from build123d import *

# Parameters (mm, degrees)
SKETCH1_R           = 1.6
SKETCH1_R_2         = 1.65
BOSS_EXTRUDE1_DEPTH = 4
FILLET2_R           = 10
FILLET3_R           = 5


with BuildPart() as part:
    # Sketch1 → Boss-Extrude1 (new body)
    with BuildSketch(Plane.XY):
        with BuildLine():
            Line((1.40773023, -0.063608297), (20.206941284, -0.063608297))
            ThreePointArc((20.206941284, -0.063608297), (20.914048066, -0.356501516), (21.206941284, -1.063608297))
            Line((21.206941284, -1.063608297), (21.206941284, -3.063608297))
            ThreePointArc((21.206941284, -3.063608297), (21.499834503, -3.770715079), (22.206941284, -4.063608297))
            Line((22.206941284, -4.063608297), (72.208519176, -4.063608297))
            ThreePointArc((72.208519176, -4.063608297), (72.915625957, -3.770715079), (73.208519176, -3.063608297))
            Line((73.208519176, -3.063608297), (73.208519176, -1.063608297))
            ThreePointArc((73.208519176, -1.063608297), (73.501412395, -0.356501516), (74.208519176, -0.063608297))
            Line((74.208519176, -0.063608297), (93.00773023, -0.063608297))
            Line((93.00773023, -0.063608297), (93.00773023, 19.936391703))
            Line((93.00773023, 19.936391703), (72.20773023, 31.430017028))
            Line((72.20773023, 31.430017028), (72.20773023, 94.442766377))
            Line((72.20773023, 94.442766377), (93.00773023, 105.936391703))
            Line((93.00773023, 105.936391703), (93.00773023, 125.936391703))
            Line((93.00773023, 125.936391703), (74.208519176, 125.936391703))
            ThreePointArc((74.208519176, 125.936391703), (73.501412395, 126.229284921), (73.208519176, 126.936391703))
            Line((73.208519176, 126.936391703), (73.208519176, 128.936391703))
            ThreePointArc((73.208519176, 128.936391703), (72.915625957, 129.643498484), (72.208519176, 129.936391703))
            Line((72.208519176, 129.936391703), (22.206941284, 129.936391703))
            ThreePointArc((22.206941284, 129.936391703), (21.499834503, 129.643498484), (21.206941284, 128.936391703))
            Line((21.206941284, 128.936391703), (21.206941284, 126.936391703))
            ThreePointArc((21.206941284, 126.936391703), (20.914048066, 126.229284921), (20.206941284, 125.936391703))
            Line((20.206941284, 125.936391703), (1.40773023, 125.936391703))
            Line((1.40773023, 125.936391703), (1.40773023, 105.936391703))
            Line((1.40773023, 105.936391703), (22.20773023, 94.442766377))
            Line((22.20773023, 94.442766377), (22.20773023, 31.430017028))
            Line((22.20773023, 31.430017028), (1.40773023, 19.936391703))
            Line((1.40773023, 19.936391703), (1.40773023, -0.063608297))
        make_face()
        with Locations((5.55773023, 4.936391703)):
            Circle(SKETCH1_R, mode=Mode.SUBTRACT)
        with Locations((14.05773023, 4.936391703)):
            Circle(SKETCH1_R, mode=Mode.SUBTRACT)
        with Locations((14.05773023, 14.936391703)):
            Circle(SKETCH1_R, mode=Mode.SUBTRACT)
        with Locations((5.55773023, 14.936391703)):
            Circle(SKETCH1_R, mode=Mode.SUBTRACT)
        with Locations(Location((69.208519176, 2.936391703, 0), (0, 0, 180))):
            Circle(SKETCH1_R, mode=Mode.SUBTRACT)
        with Locations((47.206941284, 2.936391703)):
            Circle(SKETCH1_R, mode=Mode.SUBTRACT)
        with Locations(Location((66.20773023, 54.936391703, 0), (0, 0, 180))):
            Circle(SKETCH1_R_2, mode=Mode.SUBTRACT)
        with Locations(Location((88.85773023, 14.936391703, 0), (0, 0, 180))):
            Circle(SKETCH1_R, mode=Mode.SUBTRACT)
        with Locations(Location((80.35773023, 14.936391703, 0), (0, 0, 180))):
            Circle(SKETCH1_R, mode=Mode.SUBTRACT)
        with Locations(Location((80.35773023, 4.936391703, 0), (0, 0, 180))):
            Circle(SKETCH1_R, mode=Mode.SUBTRACT)
        with Locations(Location((88.85773023, 4.936391703, 0), (0, 0, 180))):
            Circle(SKETCH1_R, mode=Mode.SUBTRACT)
        with Locations((28.20773023, 54.936391703)):
            Circle(SKETCH1_R_2, mode=Mode.SUBTRACT)
        with Locations((25.206941284, 2.936391703)):
            Circle(SKETCH1_R, mode=Mode.SUBTRACT)
        with Locations(Location((25.206941284, 122.936391703, 0), (0, 0, 180))):
            Circle(SKETCH1_R, mode=Mode.SUBTRACT)
        with Locations(Location((28.20773023, 70.936391703, 0), (0, 0, 180))):
            Circle(SKETCH1_R_2, mode=Mode.SUBTRACT)
        with Locations((88.85773023, 120.936391703)):
            Circle(SKETCH1_R, mode=Mode.SUBTRACT)
        with Locations((80.35773023, 120.936391703)):
            Circle(SKETCH1_R, mode=Mode.SUBTRACT)
        with Locations((80.35773023, 110.936391703)):
            Circle(SKETCH1_R, mode=Mode.SUBTRACT)
        with Locations((88.85773023, 110.936391703)):
            Circle(SKETCH1_R, mode=Mode.SUBTRACT)
        with Locations((66.20773023, 70.936391703)):
            Circle(SKETCH1_R_2, mode=Mode.SUBTRACT)
        with Locations(Location((47.206941284, 122.936391703, 0), (0, 0, 180))):
            Circle(SKETCH1_R, mode=Mode.SUBTRACT)
        with Locations((69.208519176, 122.936391703)):
            Circle(SKETCH1_R, mode=Mode.SUBTRACT)
        with Locations(Location((5.55773023, 110.936391703, 0), (0, 0, 180))):
            Circle(SKETCH1_R, mode=Mode.SUBTRACT)
        with Locations(Location((14.05773023, 110.936391703, 0), (0, 0, 180))):
            Circle(SKETCH1_R, mode=Mode.SUBTRACT)
        with Locations(Location((14.05773023, 120.936391703, 0), (0, 0, 180))):
            Circle(SKETCH1_R, mode=Mode.SUBTRACT)
        with Locations(Location((5.55773023, 120.936391703, 0), (0, 0, 180))):
            Circle(SKETCH1_R, mode=Mode.SUBTRACT)
    extrude(amount=BOSS_EXTRUDE1_DEPTH)

    # Fillet2
    fillet2_edges = [part.edges().sort_by_distance(p)[0] for p in [
        (1.40773023, 19.936391703, 2),
        (22.20773023, 31.430017028, 2),
        (22.20773023, 94.442766377, 2),
        (1.40773023, 105.936391703, 2),
        (93.00773023, 105.936391703, 2),
        (72.20773023, 94.442766377, 2),
        (72.20773023, 31.430017028, 2),
        (93.00773023, 19.936391703, 2),
    ]]
    fillet(fillet2_edges, radius=FILLET2_R)

    # Fillet3
    fillet3_edges = [part.edges().sort_by_distance(p)[0] for p in [
        (1.40773023, 125.936391703, 2),
        (93.00773023, 125.936391703, 2),
        (93.00773023, -0.063608297, 2),
        (1.40773023, -0.063608297, 2),
    ]]
    fillet(fillet3_edges, radius=FILLET3_R)


solid = part.part
Verification items for the finished model (mm, model axes). A direction names the side the tool comes from. Give positions to 0.01 mm unless a question says otherwise; leave off trailing zeros. Write each loop counter-clockwise with the first axis right and the second up, starting at its lowest first coordinate (ties: lowest second). Pieces come first, ordered by that corner, then holes. Notation, with made-up numbers: (-8, -12.5) - (2, -12.5) arc R23 ccw to (2, 11.5) - close; hole circle Ø4 at (-0.75, -9). An arc over 180 degrees is marked (long way). Answer as CSV lines item,"result". Start each with the question number.
1. Sectioned sample at A-A (x = 14). Record the boundary of the cut face in (y, z).
2. Thickness scan on line 1 (Y direction, x = 69.5, z = 3.15); line 2 (Y direction, x = 88, z = 3.45); line 3 (X direction, y = 123.5, z = 1.5). Record the ranges inside material, lowest first.
3. Draft check along Y on faces 4 (the face through (12.46, 15.01, 1.97)), 5 (the face through (48, 129.936, 2)), 6 (the face through (91.5, 1.36, 2.03)), 7 (the face through (24.347, 121.587, 1.972)). Enter one of: pulls with the +Y half, pulls with the -Y half, needs draft (parallel to the pull), parting line crosses it, or undercut.
4. Sectioned sample at D-D (z = 2.65). Count the separate pieces of the cut face and the enclosed holes in it, then the cut area to 3 significant figures.
5. Depth check by flat-ended pin: pin 1 (1.6 mm diameter, centred on y = -1.5, z = 1.5, fed in from -X); pin 2 (1.2 mm diameter, centred on y = 52, z = 2.5, fed in from -X); pin 3 (2 mm diameter, centred on y = 97, z = 1.5, fed in from -X). Enter the tip coordinate at first touch or a pass-through.
6. Sectioned sample at B-B (x = 47). Record the boundary of the cut face in (y, z), then the cut area to 3 significant figures.
7. Set-up check for faces 1 (the face through (13, -0.064, 2)), 2 (the face through (2.757, 19.054, 2.028)), 3 (the face through (73.633, 32.184, 2.028)): record each of +Z, -Z, +X, -X, +Y, -Y from which the full face is reachable in a straight line by a thin tool's end or side.
8. Sectioned sample at C-C (y = 41). Record the boundary of the cut face in (x, z).
Derived:
1,outline,"(-0.06, 0) - (3.34, 0) - (3.34, 4) - (-0.06, 4) - close; (6.54, 0) - (13.34, 0) - (13.34, 4) - (6.54, 4) - close; (16.54, 0) - (26.89, 0) - (26.89, 4) - (16.54, 4) - close; (98.98, 0) - (109.34, 0) - (109.34, 4) - (98.98, 4) - close; (112.54, 0) - (119.34, 0) - (119.34, 4) - (112.54, 4) - close; (122.54, 0) - (125.94, 0) - (125.94, 4) - (122.54, 4) - close"
2,line 1,"-4.06 to 1.36, 4.51 to 121.36, 124.51 to 129.94"
2,line 2,"-0.06 to 3.59, 6.29 to 13.59, 16.29 to 22.7, 103.17 to 109.59, 112.29 to 119.59, 122.29 to 125.94"
2,line 3,"2.11 to 23.71, 26.7 to 45.71, 48.7 to 67.71, 70.71 to 92.3"
3,face 4,"undercut"
3,face 5,"pulls with the +Y half"
3,face 6,"pulls with the -Y half"
3,face 7,"undercut"
4,separate pieces,"1"
4,enclosed holes,"26"
4,area,"8,630 mm²"
5,pin 1,"x = 21.14"
5,pin 2,"x = 22.21"
5,pin 3,"x = 15.77"
6,outline,"(-4.06, 0) - (1.35, 0) - (1.35, 4) - (-4.06, 4) - close; (4.52, 0) - (121.35, 0) - (121.35, 4) - (4.52, 4) - close; (124.52, 0) - (129.94, 0) - (129.94, 4) - (124.52, 4) - close"
6,area,"511 mm²"
7,face 1,"+Z, -Z, -X, -Y"
7,face 2,"+Z, -Z, -X"
7,face 3,"+Z, -Z, +X"
8,outline,"(22.21, 0) - (72.21, 0) - (72.21, 4) - (22.21, 4) - close"
